from build123d import *

# Parameters (mm, degrees)
F1_DEPTH = 38
F0_W     = 16
F0_H     = 16
F2_DEPTH = 38
F4_D     = 5
F4_DEPTH = 10
F4_TIP   = 1.5021515476
F6_D     = 6
F7_SIZE  = 1
F8_SIZE  = 1


with BuildPart() as f1:
    # F0 (on Front) → F1 (new body)
    with BuildSketch(Plane.XZ):
        with BuildLine():
            ThreePointArc((187.358939, -148.81538), (191.8844223996, -146.9408633996), (193.758939, -142.41538))
            Line((193.758939, -142.41538), (193.758939, -108.81538))
            Line((193.758939, -108.81538), (193.758939, -92.81538))
            Line((193.758939, -92.81538), (190.558939, -92.81538))
            Line((190.558939, -92.81538), (190.558939, -142.41538))
            ThreePointArc((190.558939, -142.41538), (189.6216806998, -144.6781216998), (187.358939, -145.61538))
            Line((187.358939, -145.61538), (166.758939, -145.61538))
            Line((166.758939, -145.61538), (166.758939, -148.81538))
            Line((166.758939, -148.81538), (187.358939, -148.81538))
        make_face()
    extrude(amount=-F1_DEPTH)

    # F0 (on Front) → F2 (join)
    with BuildSketch(Plane.XZ):
        with Locations((201.758939, -100.81538)):
            Rectangle(F0_W, F0_H)
    extrude(amount=-F2_DEPTH)

    # F4
    with Locations(Plane.YZ.offset(209.758939)):
        with Locations((8, -100.81538), (30, -100.81538)):
            Hole(F4_D / 2, depth=F4_DEPTH)
            with Locations((0, 0, -(F4_DEPTH + F4_TIP / 2))):  # 118° drill point
                Cone(0, F4_D / 2, F4_TIP, mode=Mode.SUBTRACT)

    # F6 (through all)
    with Locations(Plane.XY.offset(-145.61538)):
        with Locations((176.758939, 30), (176.758939, 8)):
            Hole(F6_D / 2)

    # F7
    f7_edges = [f1.edges().sort_by_distance(p)[0] for p in [
        (166.758939, 0, -147.21538),
        (166.758939, 38, -147.21538),
    ]]
    chamfer(f7_edges, length=F7_SIZE)

    # F8
    f8_edges = [f1.edges().sort_by_distance(p)[0] for p in [
        (200.158939, 0, -92.81538),
        (200.158939, 38, -92.81538),
        (201.758939, 38, -108.81538),
        (201.758939, 0, -108.81538),
    ]]
    chamfer(f8_edges, length=F8_SIZE)


solid = f1.part
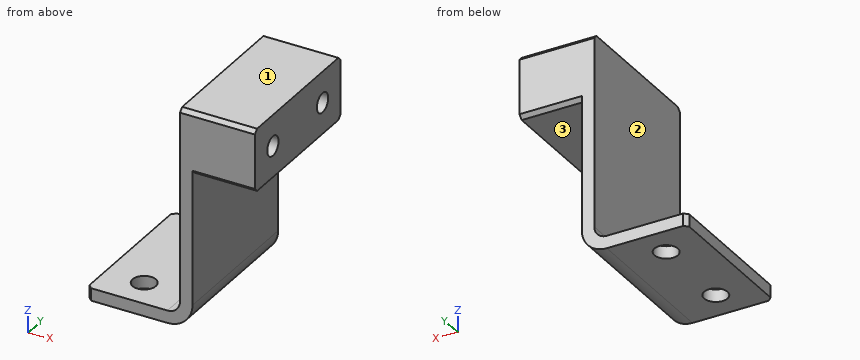
For this review, take the finished solid that the model builds, in its own axes (mm). Face numbers are marked on the shaded views. A direction names the side the tool comes from. Round coordinates to 2 decimals unless told otherwise and drop trailing zeros. Order: outer loops, then holes, each group sorted by start corner. A loop starts at its lowest first (then second) coordinate and runs counter-clockwise, first axis right, second up. Notation, with made-up numbers: M -21.5,81.5 L -11.5,81.5 A18 cw -11.5,100.5 Z; hole C 58,41.25 d3. An arc over 180 degrees is marked long. Use a Markdown table: item, result. Add a question column.
Item 1: Add section C-C, the plane z = -97.5. Give the boundary of the cut face in (x, y).
Item 2: Add section B-B, the plane y = 14. Give the boundary of the cut face in (x, z).
Item 3: Insertion check: pin 1 (6 mm diameter, centred on x = 192, y = 24, fed in from -Z); pin 2 (11.5 mm diameter, centred on y = 20, z = -115.5, fed in from -X); pin 3 (17.5 mm diameter, centred on y = 27.5, z = -121.5, fed in from +X). Each pin has a flat end and moves straight along its axis. Give the tip position at first contact, or say it passes through.
Item 4: Add section A-A, the plane x = 174.5. Give the boundary of the cut face in (y, z), then the cut area to 3 significant figures.
Item 5: To check wall thickness, follow line 1 along Z through (x, y) = (207, 30); line 2 along Z through (x, y) = (205.5, 17.5); line 3 along X through (y, z) = (22, -120). State the ranges of each line that lie inside material, in increasing order.
Item 6: Add section D-D, the plane x = 183. Give the boundary of the cut face in (y, z).
Item 7: Tool access review of the marked faces 1, 2 and 3: name each direction out of +Z, -Z, +X, -X, +Y, -Y from which nothing blocks a thin tool from reaching the whole face with its end or side.
Geometry results:
| question | item | result |
|---|---|---|
| 1 | outline | M 190.56,0 L 209.76,0 L 209.76,38 L 190.56,38 Z |
| 2 | outline | M 166.76,-148.82 L 187.36,-148.82 A6.4 ccw 193.76,-142.42 L 193.76,-108.82 L 209.76,-108.82 L 209.76,-92.82 L 190.56,-92.82 L 190.56,-142.42 A3.2 cw 187.36,-145.62 L 166.76,-145.62 Z |
| 3 | pin 1 | stops at z = -148.6 |
| 3 | pin 2 | stops at x = 190.56 |
| 3 | pin 3 | stops at x = 193.76 |
| 4 | outline | M 0,-148.82 L 6.03,-148.82 L 6.03,-145.62 L 0,-145.62 Z; M 9.97,-148.82 L 28.03,-148.82 L 28.03,-145.62 L 9.97,-145.62 Z; M 31.97,-148.82 L 38,-148.82 L 38,-145.62 L 31.97,-145.62 Z |
| 4 | area | 96.3 mm² |
| 5 | line 1 | z = -108.82 to -103.32, -98.32 to -92.82 |
| 5 | line 2 | z = -108.82 to -92.82 |
| 5 | line 3 | x = 190.56 to 193.76 |
| 6 | outline | M 0,-148.82 L 38,-148.82 L 38,-145.62 L 0,-145.62 Z |
| 7 | face 1 | +Z, +X, -X, +Y, -Y |
| 7 | face 2 | +Z, -X, +Y, -Y |
| 7 | face 3 | -Z, +X, +Y, -Y |
